Input: part model. Units: mm. Frame: model coordinates. A direction names the side the tool comes from. Round coordinates to 2 decimals unless told otherwise and drop trailing zeros. Loops run counter-clockwise (first coordinate to the right, second up) from the corner with the lowest first, then second, coordinate; pieces in that order, holes last. Notation, with made-up numbers: M 73,-26 L 113,-26 A32 ccw 113,11 Z; hole C -19,89 d10. An arc over 180 degrees is marked long. Return JSON: item names as keys, results as strings. Group by question number.
1) Contact query for flat-ended pins moving along their axis: P1, Ø2, axis at x = 9.5, y = 12, coming from the +Z side; P2, Ø2, axis at x = 2, z = 6, coming from the +Y side; P3, Ø2, axis at x = -4.5, y = 11.5, coming from the -Z side; P4, Ø6, axis at x = 13.5, y = 5.5, coming from the -Z side. Output: stop coordinate, or through.
2) Material intervals for line 1 (Y direction, x = 0.5, z = 5.5); line 2 (Z direction, x = -4, y = 19.5); line 3 (Z direction, x = 2, y = 13.25), sorted ascending. Write a range as from..to.
3) Section B-B (x = 0). Output: boundary loops of the cut face in (y, z) (3 decimals).
4) Section C-C (z = -3.5). Output: boundary loops of the cut face in (x, y), plus the area to 3 significant figures.
5) Section D-D (y = 4.5). Output: boundary loops of the cut face in (x, z) (3 decimals).
6) Access query for faces 1 (the face through (5.525, 14.489, -3.131)), 2 (the face through (0, 22.86, 7)). Directions: +Z, -Z, +X, -X, +Y, -Y. A direction counts if a zero-diameter tool reaches every point of the face in a straight line with its end or side. Return the directions, or none.
7) Section A-A (y = 11.5). Output: boundary loops of the cut face in (x, z) (3 decimals), plus the area to 3 significant figures.
8) Mould query, pull axis X, two halves, no side actions, for faces 3 (the face through (5.15, 11.27, 16.353)), 4 (the face through (-5.474, 14.489, -3.219)), 5 (the face through (0, 0, 0)). Classes: +X half, -X half, draft (parallel to the pull), parting line (faces both ways), or undercut.
from build123d import *

# Parameters (mm, degrees)
SKETCH1_R           = 17.145
BOSS_EXTRUDE1_DEPTH = 22.86
BOSS_EXTRUDE2_DEPTH = 6.35


with BuildPart() as part:
    # Sketch1 → Boss-Extrude1 (new body)
    with BuildSketch(Plane(origin=(0, 0, 0), x_dir=(1, 0, 0), z_dir=(0, 1, 0))):
        with Locations(Location((0, 0, 0), (0, 0, 270))):
            Circle(SKETCH1_R)
        Polygon((7.332348419, 0), (3.666174209, 6.35), (-3.666174209, 6.35), (-7.332348419, 0), (-3.666174209, -6.35), (3.666174209, -6.35), align=None, mode=Mode.SUBTRACT)
    extrude(amount=BOSS_EXTRUDE1_DEPTH)

    # Sketch1_2 → Boss-Extrude2 (add)
    with BuildSketch(Plane(origin=(0, 0, 0), x_dir=(1, 0, 0), z_dir=(0, 1, 0))):
        Polygon((-3.666174209, -6.35), (3.666174209, -6.35), (7.332348419, 0), (3.666174209, 6.35), (-3.666174209, 6.35), (-7.332348419, 0), align=None)
    extrude(amount=BOSS_EXTRUDE2_DEPTH)


solid = part.part
Returned:
{
 "1": {"P1": "stops at z = 14.89", "P2": "stops at y = 22.86", "P3": "stops at z = -16.78", "P4": "stops at z = -13.55"},
 "2": {"line 1": "y = 0..6.35", "line 2": "z = -16.67..-5.77, 5.77..16.67", "line 3": "z = -17.03..-6.35, 6.35..17.03"},
 "3": {"outline": "M 0,-17.145 L 22.86,-17.145 L 22.86,-6.35 L 6.35,-6.35 L 6.35,6.35 L 22.86,6.35 L 22.86,17.145 L 0,17.145 Z"},
 "4": {"outline": "M -16.78,0 L 16.78,0 L 16.78,22.86 L 5.31,22.86 L 5.31,6.35 L -5.31,6.35 L -5.31,22.86 L -16.78,22.86 Z", "area": "592 mm^2"},
 "5": {"outline": "C 0,0 d34.29"},
 "6": {"face 1": "+Y", "face 2": "+Z, -Z, +X, -X, +Y"},
 "7": {"outline": "C 0,0 d34.29; hole M -7.332,0 L -3.666,-6.35 L 3.666,-6.35 L 7.332,0 L 3.666,6.35 L -3.666,6.35 Z", "area": "784 mm^2"},
 "8": {"face 3": "parting line", "face 4": "undercut", "face 5": "draft"}
}
